```python
from build123d import *

# Parameters (mm, degrees)
SKETCH1_R           = 7.62
BOSS_EXTRUDE2_DEPTH = 10.16
SKETCH2_R           = 30.48
SKETCH2_R_2         = 19.05
CUT_EXTRUDE1_DEPTH  = 2.54
SKETCH4_R           = 30.401229143
SKETCH4_R_2         = 18.940015454
CUT_EXTRUDE3_DEPTH  = 2.54


with BuildPart() as part:
    # Sketch1 → Boss-Extrude2 (new body)
    with BuildSketch(Plane.XY):
        with BuildLine():
            ThreePointArc((-4.973047924, 37.774049218), (-9.117926809, 36.992883244), (-13.151060724, 35.758350099))
            add(Edge.make_bspline(
                [(-19.084474431, 43.633182282), (-16.926977066, 41.864131326), (-13.151060724, 35.758350099)],
                knots=[0, 0, 0, 1, 1, 1], degree=2))
            add(Edge.make_bspline(
                [(-25.068187902, 40.492687188), (-23.423529412, 44.629806533), (-19.084474431, 43.633182282)],
                knots=[0, 0, 0, 1, 1, 1], degree=2))
            add(Edge.make_bspline(
                [(-25.068187902, 40.492687188), (-24.837885701, 37.712166182), (-21.957891223, 31.136168888)],
                knots=[0, 0, 0, 1, 1, 1], degree=2))
            ThreePointArc((-21.957891223, 31.136168888), (-25.264973279, 28.518259505), (-28.262419847, 25.550843908))
            add(Edge.make_bspline(
                [(-37.175813758, 29.766266676), (-34.443325744, 29.202488866), (-28.262419847, 25.550843908)],
                knots=[0, 0, 0, 1, 1, 1], degree=2))
            add(Edge.make_bspline(
                [(-41.014668065, 24.204726066), (-41.481010519, 28.63227423), (-37.175813758, 29.766266676)],
                knots=[0, 0, 0, 1, 1, 1], degree=2))
            add(Edge.make_bspline(
                [(-41.014668065, 24.204726066), (-39.518573051, 21.849723757), (-33.912446265, 17.365367497)],
                knots=[0, 0, 0, 1, 1, 1], degree=2))
            ThreePointArc((-33.912446265, 17.365367497), (-35.624118846, 13.510446196), (-36.899199182, 9.489947298))
            add(Edge.make_bspline(
                [(-46.75062217, 9.080258097), (-44.069123581, 9.850908135), (-36.899199182, 9.489947298)],
                knots=[0, 0, 0, 1, 1, 1], degree=2))
            add(Edge.make_bspline(
                [(-47.565182054, 2.371753901), (-50.035692017, 6.075432957), (-46.75062217, 9.080258097)],
                knots=[0, 0, 0, 1, 1, 1], degree=2))
            add(Edge.make_bspline(
                [(-47.565182054, 2.371753901), (-45.146031566, 0.981772936), (-38.098068557, -0.383630312)],
                knots=[0, 0, 0, 1, 1, 1], degree=2))
            ThreePointArc((-38.098068557, -0.383630312), (-37.822208103, -4.592447518), (-37.082816668, -8.744981872))
            add(Edge.make_bspline(
                [(-45.615426449, -13.685928184), (-43.599216296, -11.757396933), (-37.082816668, -8.744981872)],
                knots=[0, 0, 0, 1, 1, 1], degree=2))
            add(Edge.make_bspline(
                [(-43.219086057, -20.0045585), (-47.12779947, -17.87321679), (-45.615426449, -13.685928184)],
                knots=[0, 0, 0, 1, 1, 1], degree=2))
            add(Edge.make_bspline(
                [(-43.219086057, -20.0045585), (-40.431078318, -20.111090232), (-33.555882474, -18.04474304)],
                knots=[0, 0, 0, 1, 1, 1], degree=2))
            ThreePointArc((-33.555882474, -18.04474304), (-31.355685291, -21.64326685), (-28.771207752, -24.976541083))
            add(Edge.make_bspline(
                [(-34.030286254, -33.31683325), (-33.141253985, -30.672224056), (-28.771207752, -24.976541083)],
                knots=[0, 0, 0, 1, 1, 1], degree=2))
            add(Edge.make_bspline(
                [(-28.972018291, -37.798067629), (-33.423496015, -37.727327965), (-34.030286254, -33.31683325)],
                knots=[0, 0, 0, 1, 1, 1], degree=2))
            add(Edge.make_bspline(
                [(-28.972018291, -37.798067629), (-26.453852274, -36.596744994), (-21.326448108, -31.572022601)],
                knots=[0, 0, 0, 1, 1, 1], degree=2))
            ThreePointArc((-21.326448108, -31.572022601), (-17.705952855, -33.735874577), (-13.868461871, -35.486275732))
            add(Edge.make_bspline(
                [(-14.649217588, -45.315253331), (-15.091029782, -42.560414288), (-13.868461871, -35.486275732)],
                knots=[0, 0, 0, 1, 1, 1], degree=2))
            add(Edge.make_bspline(
                [(-8.087810285, -46.932494981), (-12.06227242, -48.938562968), (-14.649217588, -45.315253331)],
                knots=[0, 0, 0, 1, 1, 1], degree=2))
            add(Edge.make_bspline(
                [(-8.087810285, -46.932494981), (-6.416367478, -44.698526515), (-4.211381492, -37.866532267)],
                knots=[0, 0, 0, 1, 1, 1], degree=2))
            ThreePointArc((-4.211381492, -37.866532267), (0, -38.1), (4.211381492, -37.866532267))
            add(Edge.make_bspline(
                [(8.087810285, -46.932494981), (6.416367478, -44.698526515), (4.211381492, -37.866532267)],
                knots=[0, 0, 0, 1, 1, 1], degree=2))
            add(Edge.make_bspline(
                [(14.649217588, -45.315253331), (12.06227242, -48.938562968), (8.087810285, -46.932494981)],
                knots=[0, 0, 0, 1, 1, 1], degree=2))
            add(Edge.make_bspline(
                [(14.649217588, -45.315253331), (15.091029782, -42.560414288), (13.868461871, -35.486275732)],
                knots=[0, 0, 0, 1, 1, 1], degree=2))
            ThreePointArc((13.868461871, -35.486275732), (17.705952855, -33.735874577), (21.326448108, -31.572022601))
            add(Edge.make_bspline(
                [(28.972018291, -37.798067629), (26.453852274, -36.596744994), (21.326448108, -31.572022601)],
                knots=[0, 0, 0, 1, 1, 1], degree=2))
            add(Edge.make_bspline(
                [(34.030286254, -33.31683325), (33.423496015, -37.727327965), (28.972018291, -37.798067629)],
                knots=[0, 0, 0, 1, 1, 1], degree=2))
            add(Edge.make_bspline(
                [(34.030286254, -33.31683325), (33.141253985, -30.672224056), (28.771207752, -24.976541083)],
                knots=[0, 0, 0, 1, 1, 1], degree=2))
            ThreePointArc((28.771207752, -24.976541083), (31.355685291, -21.64326685), (33.555882474, -18.04474304))
            add(Edge.make_bspline(
                [(43.219086057, -20.0045585), (40.431078318, -20.111090232), (33.555882474, -18.04474304)],
                knots=[0, 0, 0, 1, 1, 1], degree=2))
            add(Edge.make_bspline(
                [(45.615426449, -13.685928184), (47.12779947, -17.87321679), (43.219086057, -20.0045585)],
                knots=[0, 0, 0, 1, 1, 1], degree=2))
            add(Edge.make_bspline(
                [(45.615426449, -13.685928184), (43.599216296, -11.757396933), (37.082816668, -8.744981872)],
                knots=[0, 0, 0, 1, 1, 1], degree=2))
            ThreePointArc((37.082816668, -8.744981872), (37.822208103, -4.592447518), (38.098068557, -0.383630312))
            add(Edge.make_bspline(
                [(47.565182054, 2.371753901), (45.146031566, 0.981772936), (38.098068557, -0.383630312)],
                knots=[0, 0, 0, 1, 1, 1], degree=2))
            add(Edge.make_bspline(
                [(46.75062217, 9.080258097), (50.035692017, 6.075432957), (47.565182054, 2.371753901)],
                knots=[0, 0, 0, 1, 1, 1], degree=2))
            add(Edge.make_bspline(
                [(46.75062217, 9.080258097), (44.069123581, 9.850908135), (36.899199182, 9.489947298)],
                knots=[0, 0, 0, 1, 1, 1], degree=2))
            ThreePointArc((36.899199182, 9.489947298), (35.624118846, 13.510446196), (33.912446265, 17.365367497))
            add(Edge.make_bspline(
                [(41.014668065, 24.204726066), (39.518573051, 21.849723757), (33.912446265, 17.365367497)],
                knots=[0, 0, 0, 1, 1, 1], degree=2))
            add(Edge.make_bspline(
                [(37.175813758, 29.766266676), (41.481010519, 28.63227423), (41.014668065, 24.204726066)],
                knots=[0, 0, 0, 1, 1, 1], degree=2))
            add(Edge.make_bspline(
                [(37.175813758, 29.766266676), (34.443325744, 29.202488866), (28.262419847, 25.550843908)],
                knots=[0, 0, 0, 1, 1, 1], degree=2))
            ThreePointArc((28.262419847, 25.550843908), (25.264973279, 28.518259505), (21.957891223, 31.136168888))
            add(Edge.make_bspline(
                [(25.068187902, 40.492687188), (24.837885701, 37.712166182), (21.957891223, 31.136168888)],
                knots=[0, 0, 0, 1, 1, 1], degree=2))
            add(Edge.make_bspline(
                [(19.084474431, 43.633182282), (23.423529412, 44.629806533), (25.068187902, 40.492687188)],
                knots=[0, 0, 0, 1, 1, 1], degree=2))
            add(Edge.make_bspline(
                [(19.084474431, 43.633182282), (16.926977066, 41.864131326), (13.151060724, 35.758350099)],
                knots=[0, 0, 0, 1, 1, 1], degree=2))
            ThreePointArc((13.151060724, 35.758350099), (9.117926809, 36.992883244), (4.973047924, 37.774049218))
            add(Edge.make_bspline(
                [(3.378887996, 47.504261665), (4.467138065, 44.935205816), (4.973047924, 37.774049218)],
                knots=[0, 0, 0, 1, 1, 1], degree=2))
            add(Edge.make_bspline(
                [(-3.378887996, 47.504261665), (0, 50.403188007), (3.378887996, 47.504261665)],
                knots=[0, 0, 0, 1, 1, 1], degree=2))
            add(Edge.make_bspline(
                [(-3.378887996, 47.504261665), (-4.467138065, 44.935205816), (-4.973047924, 37.774049218)],
                knots=[0, 0, 0, 1, 1, 1], degree=2))
        make_face()
        Circle(SKETCH1_R, mode=Mode.SUBTRACT)
    extrude(amount=BOSS_EXTRUDE2_DEPTH)

    # Sketch2 → Cut-Extrude1 (cut)
    with BuildSketch(Plane(origin=(0, 0, 0), x_dir=(-1, 0, 0), z_dir=(0, 0, -1))):
        Circle(SKETCH2_R)
        Circle(SKETCH2_R_2, mode=Mode.SUBTRACT)
    extrude(amount=-CUT_EXTRUDE1_DEPTH, mode=Mode.SUBTRACT)

    # Sketch4 → Cut-Extrude3 (cut)
    with BuildSketch(Plane.XY.offset(10.16)):
        Circle(SKETCH4_R)
        Circle(SKETCH4_R_2, mode=Mode.SUBTRACT)
    extrude(amount=-CUT_EXTRUDE3_DEPTH, mode=Mode.SUBTRACT)


solid = part.part
```
Input: part model. Units: mm. Frame: model coordinates. A direction names the side the tool comes from. Round coordinates to 2 decimals unless told otherwise and drop trailing zeros.
1) Pull-direction query (X, two-part tool) for faces 6 (the cylindrical face through (-37.83, -4.53, 5.01)), 7 (the flat face through (8, 0, 0)), 8 (the flat face through (0, -20, 2.54)); classes: released by +X, released by -X, zero draft, split by the parting line, or undercut.
Ans:
face 6: released by -X
face 7: zero draft
face 8: undercut
2) Pin query (flat end, axial travel): pin 1 (4 mm diameter, centred on y = 19.5, z = 6.5, fed in from -X); pin 2 (5 mm diameter, centred on x = -37, z = 3.5, fed in from +Y); pin 3 (18.5 mm diameter, centred on x = -4, y = -12, fed in from -Z). Return the tip coordinate at first contact, or that it passes through.
Ans:
pin 1: stops at x = -38.68
pin 2: stops at y = 29.77
pin 3: stops at z = 0
3) Section query A-A on z = 1.25. Count the separate pieces of the cut face and the enclosed holes in it, plus the area to 3 significant figures.
Ans:
separate pieces: 2
enclosed holes: 2
area: 3,770 mm2
4) Material intervals for line 1 (Y direction, x = 0, z = 0.8); line 2 (Y direction, x = 0, z = 9.3); line 3 (Y direction, x = 17, z = 9), sorted ascending.
Ans:
line 1: y = -38.1 to -30.48, -19.05 to -7.62, 7.62 to 19.05, 30.48 to 48.95
line 2: y = -38.1 to -30.4, -18.94 to -7.62, 7.62 to 18.94, 30.4 to 48.95
line 3: y = -34.1 to -25.2, -8.35 to 8.35, 25.2 to 41.4
5) Set-up query: faces 1 (the cylindrical face through (-31.39, -21.59, 5.01)), 2 (the cylindrical face through (6.607, -29.755, 1.252)), 3 (the flat face through (13, 14, 7.62)), 4 (the flat face through (7, 30, 0)), 5 (the cylindrical face through (-9.061, 37.007, 5.009)). Return all of +Z, -Z, +X, -X, +Y, -Y with unobstructed straight access to the full face (end or side cutting, diameter ignored); none if empty.
Ans:
face 1: +Z, -Z
face 2: -Z
face 3: +Z
face 4: -Z, +X, -X, +Y, -Y
face 5: +Z, -Z, +Y
